Part model, mm, in its own coordinate system. Face numbers are marked on the shaded views. A direction names the side the tool comes from. Round coordinates to 2 decimals unless told otherwise and drop trailing zeros. Loops run counter-clockwise (first coordinate to the right, second up) from the corner with the lowest first, then second, coordinate; pieces in that order, holes last.
from build123d import *

# Parameters (mm, degrees)
F1_DEPTH = 6.35
F2_W     = 6.35
F2_H     = 2.54
F3_DEPTH = 15.24
F5_DEPTH = 2.54


with BuildPart() as f1:
    # F0 (on Top) → F1 (new body)
    with BuildSketch(Plane.XY):
        Polygon((-12.7, -50.8), (-6.35, -50.8), (0, -50.8), (0, 0), (50.8, 0), (50.8, 50.8), (44.45, 50.8), (44.45, 6.35), (-57.15, 6.35), (-57.15, 50.8), (-63.5, 50.8), (-63.5, 0), (-12.7, 0), align=None)
    extrude(amount=F1_DEPTH)

    # F2 (on face) → F3 (join)
    with BuildSketch(Plane(origin=(0, 0, 0), x_dir=(1, 0, 0), z_dir=(0, 0, -1))):
        Polygon((0, 25.4), (-6.35, 25.4), (-12.7, 25.4), (-12.7, 22.86), (0, 22.86), align=None)
        with Locations((-9.525, 49.53)):
            Rectangle(F2_W, F2_H)
        with Locations((-3.175, 49.53)):
            Rectangle(F2_W, F2_H)
    extrude(amount=F3_DEPTH)

    # F4 (on face) → F5 (cut, through all)
    with BuildSketch(Plane.XZ.offset(50.8)):
        Polygon((-11.8491, -10.794907), (-6.35, -13.969814), (-0.8509, -10.794907), (-0.8509, -4.445093), (-6.35, -1.270186), (-11.8491, -4.445093), align=None)
    extrude(amount=-F5_DEPTH, mode=Mode.SUBTRACT)


solid = f1.part
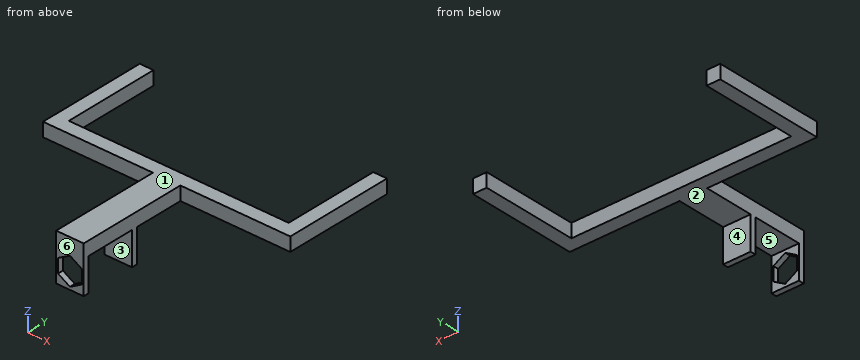
1) Tool access for the marked faces 1 and 2: list every direction of +Z, -Z, +X, -X, +Y, -Y with a clear straight run to the whole face (end or side of a thin tool).
Values:
face 1: +Z, +X, -X, +Y, -Y
face 2: -Z, +X, -X, +Y
2) Mould opens along Y. For the marked faces 3, 4, 5 and 6 say: released by +Y, released by -Y, zero draft, split by the parting line, or undercut.
Values:
face 3: undercut
face 4: released by +Y
face 5: undercut
face 6: released by -Y
3) Slice it at D-D, the plane z = 2.5. Give the cut face in (x, y), then the cut area to 3 significant figures.
Values:
outline: (-63.5, 0) - (-12.7, 0) - (-12.7, -50.8) - (0, -50.8) - (0, 0) - (50.8, 0) - (50.8, 50.8) - (44.45, 50.8) - (44.45, 6.35) - (-57.15, 6.35) - (-57.15, 50.8) - (-63.5, 50.8) - close
area: 1,940 mm2
4) Drop flat-ended pins along their axis: pin 1 Ø5 at (x, z) = (-7.5, 2) entering from +Y; pin 2 Ø4 at (x, y) = (-6.5, -34.5) entering from -Z; pin 3 Ø11 at (y, z) = (-21.5, -7) entering from -X. Give the stop position or say it passes through.
Values:
pin 1: stops at y = 6.35
pin 2: stops at z = 0
pin 3: stops at x = -12.7
5) Slice it at C-C, the plane x = -9.5. Give the cut face in (y, z).
Values:
outline: (-50.8, -15.24) - (-48.26, -15.24) - (-48.26, -12.15) - (-50.8, -12.15) - close; (-50.8, -3.09) - (-48.26, -3.09) - (-48.26, 0) - (-25.4, 0) - (-25.4, -15.24) - (-22.86, -15.24) - (-22.86, 0) - (6.35, 0) - (6.35, 6.35) - (-50.8, 6.35) - close
6) Slice it at B-B, the plane y = 34.5. Give the cut face in (x, z), then the cut area to 3 significant figures.
Values:
outline: (-63.5, 0) - (-57.15, 0) - (-57.15, 6.35) - (-63.5, 6.35) - close; (44.45, 0) - (50.8, 0) - (50.8, 6.35) - (44.45, 6.35) - close
area: 80.6 mm2
7) Slice it at A-A, the plane z = -8. Give the cut face in (x, y), then the cut area to 3 significant figures.
Values:
outline: (-12.7, -50.8) - (-11.85, -50.8) - (-11.85, -48.26) - (-12.7, -48.26) - close; (-12.7, -25.4) - (0, -25.4) - (0, -22.86) - (-12.7, -22.86) - close; (-0.85, -50.8) - (0, -50.8) - (0, -48.26) - (-0.85, -48.26) - close
area: 36.6 mm2
8) Wall check: line 1 along X through (y, z) = (42, 4.5); line 2 along Z through (x, y) = (44.5, 9); line 3 along X through (y, z) = (-13.5, 5). Give the ranges that are in metal, low to high.
Values:
line 1: x = -63.5 to -57.15, 44.45 to 50.8
line 2: z = 0 to 6.35
line 3: x = -12.7 to 0
